from build123d import *

# Parameters (mm, degrees)
SKETCH1_R           = 47.75
SKETCH1_R_2         = 42.75
BOSS_EXTRUDE1_DEPTH = 1.25
BOSS_EXTRUDE2_START = 5
SKETCH2_R           = 47.75
SKETCH2_R_2         = 2.25
BOSS_EXTRUDE2_DEPTH = 5
SKETCH3_R           = 3.875
CUT_EXTRUDE1_DEPTH  = 4.75
BOSS_EXTRUDE3_START = 10
SKETCH4_W           = 12.7
SKETCH4_H           = 20
SKETCH4_R           = 2.25
BOSS_EXTRUDE3_DEPTH = 10
FILLET1_R           = 10
FILLET2_R           = 1


with BuildPart() as part:
    # Sketch1 → Boss-Extrude1 (new body)
    with BuildSketch(Plane(origin=(0, 0, 0), x_dir=(0, 1, 0), z_dir=(0, 0, 1))):
        with Locations(Location((0, 0, 0), (0, 0, 270))):
            Circle(SKETCH1_R)
        with Locations(Location((0, 0, 0), (0, 0, 270))):
            Circle(SKETCH1_R_2, mode=Mode.SUBTRACT)
    extrude(amount=BOSS_EXTRUDE1_DEPTH)

    # Sketch2 → Boss-Extrude2 (add)
    with BuildSketch(Plane(origin=(0, 0, 0), x_dir=(1, 0, 0), z_dir=(0, 0, -1)).offset(BOSS_EXTRUDE2_START)):
        with Locations(Location((0, 0, 0), (0, 0, 180))):
            Circle(SKETCH2_R)
        with Locations(Location((0, 5, 0), (0, 0, 180))):
            Circle(SKETCH2_R_2, mode=Mode.SUBTRACT)
        with Locations(Location((0, -5, 0), (0, 0, 180))):
            Circle(SKETCH2_R_2, mode=Mode.SUBTRACT)
    extrude(amount=-BOSS_EXTRUDE2_DEPTH)

    # Sketch3 → Cut-Extrude1 (cut)
    with BuildSketch(Plane.XY):
        with Locations((0, 5)):
            Circle(SKETCH3_R)
        with Locations((0, -5)):
            Circle(SKETCH3_R)
    extrude(amount=-CUT_EXTRUDE1_DEPTH, mode=Mode.SUBTRACT)

    # Sketch4 → Boss-Extrude3 (add)
    with BuildSketch(Plane(origin=(0, 0, -5), x_dir=(1, 0, 0), z_dir=(0, 0, -1)).offset(BOSS_EXTRUDE3_START)):
        Rectangle(SKETCH4_W, SKETCH4_H)
        with Locations((0, 5)):
            Circle(SKETCH4_R, mode=Mode.SUBTRACT)
        with Locations((0, -5)):
            Circle(SKETCH4_R, mode=Mode.SUBTRACT)
    extrude(amount=-BOSS_EXTRUDE3_DEPTH)

    # Fillet1
    fillet1_edges = [part.edges().sort_by_distance(p)[0] for p in [
        (0, -10, -5),
        (-6.35, 0, -5),
        (0, 10, -5),
        (6.35, 0, -5),
    ]]
    fillet(fillet1_edges, radius=FILLET1_R - 0.0001)  # a hair under: the kernel refuses the full size

    # Fillet2
    fillet2_edges = [part.edges().sort_by_distance(p)[0] for p in [
        (47.75, 0, -5),
        (-47.75, 0, 1.25),
    ]]
    fillet(fillet2_edges, radius=FILLET2_R)


solid = part.part
Source: CAD feature listing. Evaluate the final solid. Frame: model axes, mm. A direction names the side the tool comes from. Round coordinates to 2 decimals unless told otherwise and drop trailing zeros.
Q1. First-contact query: P1, Ø2.5, axis at x = 0, y = -5, coming from the -Z side; P2, Ø8, axis at x = 33.5, z = -8.5, coming from the +Y side; P3, Ø10, axis at x = -0.5, y = -20.5, coming from the -Z side; P4, Ø10, axis at x = 0, y = -5, coming from the +Z side. Flat tips, straight axial feed; report the tip coordinate or a pass-through.
Q2. Section A-A, the plane x = 0. State how many separate pieces and enclosed holes the cut face has, plus the area to 3 significant figures.
Q3. Mould query, pull axis Y, two halves, no side actions, for faces 1 (the face through (0.148, 2.755, -9.947)), 2 (the face through (10.7, -0.28, -6.75)), 3 (the face through (1, 1, 0)), 4 (the face through (0, -14, -7)). Classes: pulls with the +Y half, pulls with the -Y half, needs draft (parallel to the pull), parting line crosses it, or undercut.
Q4. Access query for faces 5 (the face through (0, 0, -15)), 6 (the face through (-20, 1, -5)), 7 (the face through (2, -7, -4.75)). Directions: +Z, -Z, +X, -X, +Y, -Y. A direction counts if a zero-diameter tool reaches every point of the face in a straight line with its end or side. Return the directions, or none.
Q5. Ray query, line 1 (Y direction, x = 0, z = -1.9) (3 decimals); line 2 (Y direction, x = -1.5, z = 0.75); line 3 (Z direction, x = -6, y = -40). Return the intervals inside material, ascending.
Solutions:
1. P1: passes through
1. P2: stops at y = 34.93
1. P3: stops at z = -6.07
1. P4: stops at z = 0
2. separate pieces: 3
2. enclosed holes: 0
2. area: 566 mm2
3. face 1: undercut
3. face 2: needs draft
3. face 3: undercut
3. face 4: pulls with the -Y half
4. face 5: -Z, +X, -X, +Y, -Y
4. face 6: -Z
4. face 7: +Z
5. line 1: y = -47.75 to -8.875, -1.125 to 1.125, 8.875 to 47.75
5. line 2: y = -47.59 to -42.72, 42.72 to 47.59
5. line 3: z = -5 to 0
